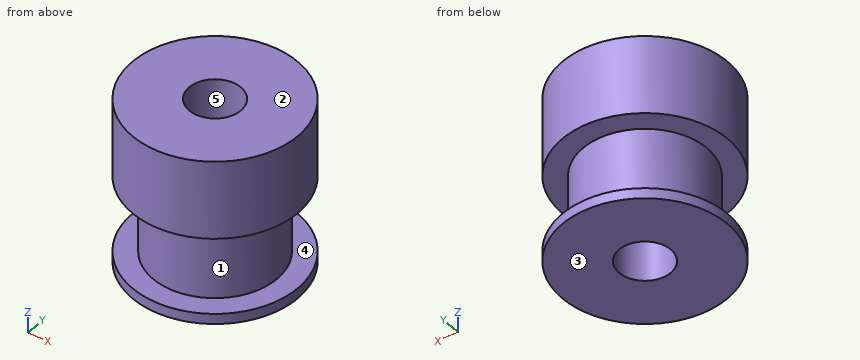
```python
from build123d import *

# Parameters (mm, degrees)
SKETCH_1_R          = 8
EXTRUDE_1_DEPTH     = 1
SKETCH_2_R          = 6
EXTRUDE_2_DEPTH     = 7.4
SKETCH_3_R          = 8
EXTRUDE_3_DEPTH     = 7.6
SKETCH_4_R          = 2.5
CUT_EXTRUDE_1_DEPTH = 17


with BuildPart() as part:
    # 草图1 → 凸台-拉伸1 (new body)
    with BuildSketch(Plane.XY):
        Circle(SKETCH_1_R)
    extrude(amount=EXTRUDE_1_DEPTH)

    # 草图2 → 凸台-拉伸2 (add)
    with BuildSketch(Plane.XY.offset(1)):
        Circle(SKETCH_2_R)
    extrude(amount=EXTRUDE_2_DEPTH)

    # 草图3 → 凸台-拉伸3 (add)
    with BuildSketch(Plane.XY.offset(8.4)):
        Circle(SKETCH_3_R)
    extrude(amount=EXTRUDE_3_DEPTH)

    # 草图4 → 切除-拉伸1 (cut, through all)
    with BuildSketch(Plane(origin=(0, 0, 0), x_dir=(-1, 0, 0), z_dir=(0, 0, -1))):
        Circle(SKETCH_4_R)
    extrude(amount=-CUT_EXTRUDE_1_DEPTH, mode=Mode.SUBTRACT)


solid = part.part
```
Can you work these out from the model? Positions are in its coordinate system, mm. Face numbers are marked on the shaded views. A direction names the side the tool comes from. Round coordinates to 2 decimals unless told otherwise and drop trailing zeros. Loops run counter-clockwise (first coordinate to the right, second up) from the corner with the lowest first, then second, coordinate; pieces in that order, holes last. Notation, with made-up numbers: M 60.25,83.25 L 106.25,83.25 A11 cw 106.25,102.25 Z; hole C 68.5,33 d2. An arc over 180 degrees is marked long. Answer in a Markdown table with one row per item.
1. Thinking about a two-plate mould opening in Z: for the marked faces 1, 2 and 3, which applies, pulls with the +Z half, pulls with the -Z half, needs draft (parallel to the pull), parting line crosses it, or undercut?
Established:
| item | result |
|---|---|
| face 1 | undercut |
| face 2 | pulls with the +Z half |
| face 3 | pulls with the -Z half |
2. On a 3-axis mill with a long thin cutter (end or side, diameter ignored), from which of +Z, -Z, +X, -X, +Y, -Y can I reach the whole of each face in a straight line? I mean the marked faces 4 and 5. Say none if no direction works.
Established:
| item | result |
|---|---|
| face 4 | none |
| face 5 | +Z, -Z |
3. If we section it at C-C, the plane z = 11.75: Please give me the cut outline in (x, y).
Established:
| item | result |
|---|---|
| outline | C 0,0 d16; hole C 0,0 d5 |
4. I'm going to push flat-ended pins straight in: pin 1 Ø1.5 at (x, z) = (-5, 9) entering from +Y; pin 2 Ø6.5 at (x, y) = (0, 0) entering from +Z; pin 3 Ø4 at (y, z) = (-4, 7) entering from +X; pin 4 Ø1.5 at (y, z) = (6, 2) entering from -X. Where does each tip first touch, or does it pass through?
Established:
| item | result |
|---|---|
| pin 1 | y = 6.78 |
| pin 2 | z = 16 |
| pin 3 | x = 7.58 |
| pin 4 | x = -2.9 |
5. If we section it at D-D, the plane y = -5: Please give me the cut outline in (x, z) (3 decimals).
Established:
| item | result |
|---|---|
| outline | M -6.245,0 L 6.245,0 L 6.245,1 L 3.317,1 L 3.317,8.4 L 6.245,8.4 L 6.245,16 L -6.245,16 L -6.245,8.4 L -3.317,8.4 L -3.317,1 L -6.245,1 Z |
6. If we section it at A-A, the plane x = 0: Please give me the cut outline in (y, z), plus the area to 3 significant figures.
Established:
| item | result |
|---|---|
| outline | M -8,0 L -2.5,0 L -2.5,16 L -8,16 L -8,8.4 L -6,8.4 L -6,1 L -8,1 Z; M 2.5,0 L 8,0 L 8,1 L 6,1 L 6,8.4 L 8,8.4 L 8,16 L 2.5,16 Z |
| area | 146 mm² |
7. Please list where these lines run through material, in increasing order: line 1 (Z direction, x = 0.75, y = 6); line 2 (Y direction, x = 0, z = 11.5); line 3 (Y direction, x = 0, z = 3). Write a range as from..to.
Established:
| item | result |
|---|---|
| line 1 | 0..1, 8.4..16 |
| line 2 | -8..-2.5, 2.5..8 |
| line 3 | -6..-2.5, 2.5..6 |
